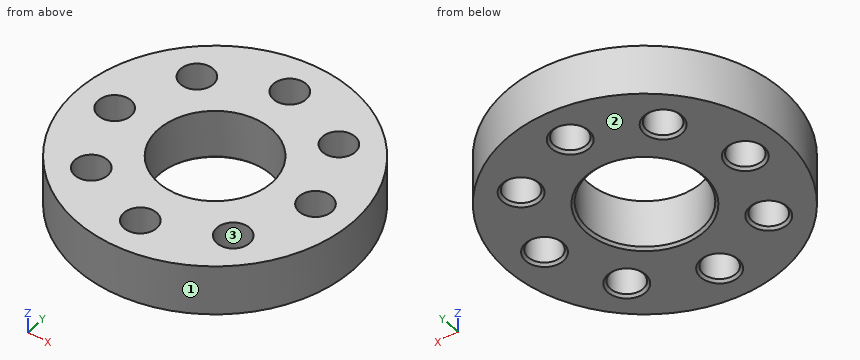
```python
from build123d import *

# Parameters (mm, degrees)
SKETCH_R        = 11
PAD_DEPTH       = 4
SKETCH002_R     = 4.5
SKETCH002_R_2   = 1.3
POCKET001_DEPTH = 10
CHAMFER_SIZE    = 0.2


with BuildPart() as part:
    # Sketch → Pad (new body)
    with BuildSketch(Plane.XY):
        Circle(SKETCH_R)
    extrude(amount=PAD_DEPTH)

    # Sketch002 → Pocket001 (cut)
    with BuildSketch(Plane.XY.offset(6)):
        Circle(SKETCH002_R)
        with Locations((0, 8)):
            Circle(SKETCH002_R_2)
        with Locations((5.656854, 5.656854)):
            Circle(SKETCH002_R_2)
        with Locations((8, 0)):
            Circle(SKETCH002_R_2)
        with Locations((5.656854, -5.656854)):
            Circle(SKETCH002_R_2)
        with Locations((0, -8)):
            Circle(SKETCH002_R_2)
        with Locations((-5.656854, -5.656854)):
            Circle(SKETCH002_R_2)
        with Locations((-8, 0)):
            Circle(SKETCH002_R_2)
        with Locations((-5.656854, 5.656854)):
            Circle(SKETCH002_R_2)
    extrude(amount=-POCKET001_DEPTH, mode=Mode.SUBTRACT)

    # Chamfer
    chamfer_edges = [part.edges().sort_by_distance(p)[0] for p in [
        (4.356854, 5.656854, 0),
        (-6.956854, 5.656854, 0),
        (4.356854, -5.656854, 0),
        (-9.3, 0, 0),
        (-6.956854, -5.656854, 0),
        (-1.3, -8, 0),
        (-1.3, 8, 0),
        (-4.5, 0, 0),
        (6.7, 0, 0),
    ]]
    chamfer(chamfer_edges, length=CHAMFER_SIZE)


solid = part.part
```
The listing builds one solid part. Answer for the finished solid, in the listing's coordinates (mm). Face numbers are marked on the shaded views. Coordinates: 2 decimals unless noted, no trailing zeros. Loops run counter-clockwise (first coordinate to the right, second up) from the corner with the lowest first, then second, coordinate; pieces in that order, holes last. Notation, with made-up numbers: M 55,35 L 86,35 A30 ccw 86,65 Z; hole C -13.5,-19 d5. An arc over 180 degrees is marked long. Answer as a JSON object with one key per item and string values. Group by question number.
Item 1: Section C-C (z = 1.05) is taken. Give the number of separate pieces and of enclosed holes in the cut face, and give its area (3 significant figures).
Item 2: Determine the mould class of the marked faces 1, 2 and 3 for opening direction Y: +Y half, -Y half, draft (parallel to the pull), parting line (faces both ways), or undercut.
Item 3: Section D-D (y = -8) is taken. Write down the section's boundary in (x, z).
Item 4: Section A-A (x = 0) is taken. Write down the section's boundary in (y, z), and give its area (3 significant figures).
Item 5: Each of these flat-tipped pins is pushed along its axis until it touches: P1, Ø1.6, axis at x = -5.66, y = 5.66, coming from the +Z side; P2, Ø1.5, axis at y = 4, z = 3, coming from the +X side; P3, Ø1.5, axis at y = 4.5, z = 1.5, coming from the -X side. Where does it stop, or does it pass through?
Item 6: Consider L1, parallel to Y at x = 0, z = 2.35; L2, parallel to Y at x = -1, z = 2.9; L3, parallel to Y at x = 3, z = 2.5. Determine where each line is inside the solid, lowest interval first.
Solved:
{
 "1": {"separate pieces": "1", "enclosed holes": "9", "area": "274 mm2"},
 "2": {"face 1": "parting line", "face 2": "draft", "face 3": "undercut"},
 "3": {"outline": "M -7.55,0 L -1.5,0 L -1.3,0.2 L -1.3,4 L -7.55,4 Z; M 1.3,0.2 L 1.5,0 L 7.55,0 L 7.55,4 L 1.3,4 Z"},
 "4": {"outline": "M -11,0 L -9.5,0 L -9.3,0.2 L -9.3,4 L -11,4 Z; M -6.7,0.2 L -6.5,0 L -4.7,0 L -4.5,0.2 L -4.5,4 L -6.7,4 Z; M 4.5,0.2 L 4.7,0 L 6.5,0 L 6.7,0.2 L 6.7,4 L 4.5,4 Z; M 9.3,0.2 L 9.5,0 L 11,0 L 11,4 L 9.3,4 Z", "area": "31.1 mm2"},
 "5": {"P1": "passes through", "P2": "stops at x = 10.51", "P3": "stops at x = -10.34"},
 "6": {"L1": "y = -11 to -9.3, -6.7 to -4.5, 4.5 to 6.7, 9.3 to 11", "L2": "y = -10.95 to -8.83, -7.17 to -4.39, 4.39 to 7.17, 8.83 to 10.95", "L3": "y = -10.58 to -3.35, 3.35 to 10.58"}
}
